```python
from build123d import *

# Parameters (mm, degrees)
SKETCH1_W             = 20
SKETCH1_H             = 20
SKETCH1_W_2           = 18
SKETCH1_H_2           = 18
F_20_X_20_X_2_1_DEPTH = 364.53
SKETCH_2_R            = 2.5
CUT_EXTRUDE_1_DEPTH   = 366.215170687


with BuildPart() as part:
    # Sketch1 → 方形管 20 X 20 X 2(1) (new body)
    with BuildSketch(Plane(origin=(0, 0, 0), x_dir=(-1, 0, 0), z_dir=(0, 1, 0))):
        Rectangle(SKETCH1_W, SKETCH1_H)
        Rectangle(SKETCH1_W_2, SKETCH1_H_2, mode=Mode.SUBTRACT)
    extrude(amount=F_20_X_20_X_2_1_DEPTH)

    # 草图2 → 切除-拉伸1 (cut, through all)
    with BuildSketch(Plane.XY.offset(10)):
        with Locations((0, 10)):
            Circle(SKETCH_2_R)
        with Locations((0, 22.5)):
            Circle(SKETCH_2_R)
        with Locations((0, 35)):
            Circle(SKETCH_2_R)
    extrude(amount=-CUT_EXTRUDE_1_DEPTH, mode=Mode.SUBTRACT)


solid = part.part
```
Verification items for the finished model (mm, model axes). A direction names the side the tool comes from. Coordinates: 2 decimals unless noted, no trailing zeros. Write each loop counter-clockwise with the first axis right and the second up, starting at its lowest first coordinate (ties: lowest second). Pieces come first, ordered by that corner, then holes. Notation, with made-up numbers: M -30.75,58 L 14.25,58 A22 cw 14.25,69 Z; hole C 22.25,72 d8. An arc over 180 degrees is marked long. Answer as a JSON object with one key per item and string values. Group by question number.
(1) Cross-section at B-B, the plane z = 6. Record the cut outline in (x, y), and give its area (3 significant figures).
(2) Tool access check on faces 1 (the face through (10, 180, 0)), 2 (the face through (-9, 180, 0)). Record the directions out of +Z, -Z, +X, -X, +Y, -Y that give a thin tool (end or side, any length) a straight path to the whole face; none if there is none.
(3) Cross-section at A-A, the plane x = 5.5. Record the cut outline in (y, z).
(4) Release check for a two-part mould opening along Z. For faces 3 (the face through (0.8, 364.53, -9.6)), 4 (the face through (0, 180, -9)), 5 (the face through (0, 180, 10)), 6 (the face through (0, 180, -10)) record: +Z half, -Z half, draft (parallel to the pull), parting line (faces both ways), or undercut.
(5) Gauge pin test, flat end, axial feed: pin 1 (4 mm diameter, centred on x = 0, y = 35, fed in from -Z) (3 decimals). Record the tip position at first contact, or that the pin passes through.
(6) Cross-section at C-C, the plane y = 104. Record the cut outline in (x, z), and give its area (3 significant figures).
(7) Material ranges on line 1 (Y direction, x = 0, z = -9.3); line 2 (X direction, y = 242, z = 8.5), recorded low to high.
Reply:
{
 "1": {"outline": "M -10,0 L -9,0 L -9,364.53 L -10,364.53 Z; M 9,0 L 10,0 L 10,364.53 L 9,364.53 Z", "area": "729 mm²"},
 "2": {"face 1": "+Z, -Z, +X, +Y, -Y", "face 2": "+Y, -Y"},
 "3": {"outline": "M 0,-10 L 364.53,-10 L 364.53,-9 L 0,-9 Z; M 0,9 L 364.53,9 L 364.53,10 L 0,10 Z"},
 "4": {"face 3": "draft", "face 4": "undercut", "face 5": "+Z half", "face 6": "-Z half"},
 "5": {"pin 1": "through"},
 "6": {"outline": "M -10,-10 L 10,-10 L 10,10 L -10,10 Z; hole M -9,-9 L 9,-9 L 9,9 L -9,9 Z", "area": "76.0 mm²"},
 "7": {"line 1": "0 to 7.5, 12.5 to 20, 25 to 32.5, 37.5 to 364.53", "line 2": "-10 to -9, 9 to 10"}
}
